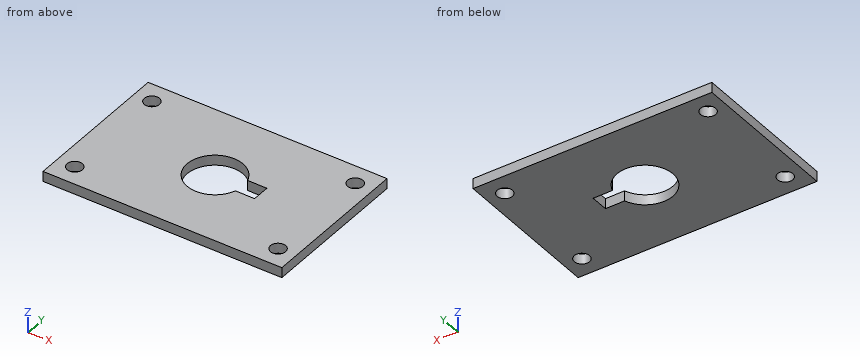
from build123d import *

# Parameters (mm, degrees)
SKETCH_1_W          = 47
SKETCH_1_H          = 30
EXTRUDE_1_DEPTH     = 2
SKETCH_2_R          = 5.5
CUT_EXTRUDE_1_DEPTH = 56.794264938
SKETCH_3_W          = 7
SKETCH_3_H          = 3.5
CUT_EXTRUDE_2_DEPTH = 56.794264938
SKETCH_4_R          = 1.5
CUT_EXTRUDE_3_DEPTH = 56.794264938


with BuildPart() as part:
    # Эскиз1 → Бобышка-Вытянуть1 (new body)
    with BuildSketch(Plane.XY):
        with Locations((23.5, 15)):
            Rectangle(SKETCH_1_W, SKETCH_1_H)
    extrude(amount=EXTRUDE_1_DEPTH)

    # Эскиз2 → Вырез-Вытянуть1 (cut, through all)
    with BuildSketch(Plane.XY.offset(2)):
        with Locations((23.5, 15)):
            Circle(SKETCH_2_R)
    extrude(amount=-CUT_EXTRUDE_1_DEPTH, mode=Mode.SUBTRACT)

    # Эскиз3 → Вырез-Вытянуть2 (cut, through all)
    with BuildSketch(Plane.XY.offset(2)):
        with Locations((29, 15)):
            Rectangle(SKETCH_3_W, SKETCH_3_H)
    extrude(amount=-CUT_EXTRUDE_2_DEPTH, mode=Mode.SUBTRACT)

    # Эскиз4 → Вырез-Вытянуть3 (cut, through all)
    with BuildSketch(Plane.XY.offset(2)):
        with Locations((3.5, 4)):
            Circle(SKETCH_4_R)
        with Locations((43.5, 4)):
            Circle(SKETCH_4_R)
        with Locations((43.5, 26)):
            Circle(SKETCH_4_R)
        with Locations((3.5, 26)):
            Circle(SKETCH_4_R)
    extrude(amount=-CUT_EXTRUDE_3_DEPTH, mode=Mode.SUBTRACT)


solid = part.part
CAD build for the part. Positions are in the model's coordinates, mm. Coordinates: 2 decimals unless noted, no trailing zeros. Order: outer loops, then holes, each group sorted by start corner. A loop starts at its lowest first (then second) coordinate and runs counter-clockwise, first axis right, second up.
Item 1: Band-saw the part on A-A on x = 43.5. List the corners of the cut face in (y, z), plus the area to 3 significant figures.
Check sheet entries:
outline: (0, 0) - (2.5, 0) - (2.5, 2) - (0, 2) - close; (5.5, 0) - (24.5, 0) - (24.5, 2) - (5.5, 2) - close; (27.5, 0) - (30, 0) - (30, 2) - (27.5, 2) - close
area: 48.0 mm2
Item 2: Band-saw the part on B-B on y = 4. List the corners of the cut face in (x, z).
Check sheet entries:
outline: (0, 0) - (2, 0) - (2, 2) - (0, 2) - close; (5, 0) - (42, 0) - (42, 2) - (5, 2) - close; (45, 0) - (47, 0) - (47, 2) - (45, 2) - close
Item 3: Band-saw the part on D-D on z = 1.7. List the corners of the cut face in (x, y), plus the area to 3 significant figures.
Check sheet entries:
outline: (0, 0) - (47, 0) - (47, 30) - (0, 30) - close; hole circle Ø3 at (3.5, 4); hole circle Ø3 at (3.5, 26); hole (28.71, 13.25) - (32.5, 13.25) - (32.5, 16.75) - (28.71, 16.75) arc R5.5 ccw (long way) to start; hole circle Ø3 at (43.5, 4); hole circle Ø3 at (43.5, 26)
area: 1,270 mm2
Item 4: Band-saw the part on C-C on x = 23.5. List the corners of the cut face in (y, z).
Check sheet entries:
outline: (0, 0) - (9.5, 0) - (9.5, 2) - (0, 2) - close; (20.5, 0) - (30, 0) - (30, 2) - (20.5, 2) - close
Item 5: Drill centre lines: L1, parallel to Y at x = 43.5, z = 1.3; L2, parallel to Y at x = 2.5, z = 1.45; L3, parallel to Y at x = 29.5, z = 0.75. Where is each one in solid material? Low to high.
Check sheet entries:
L1: y = 0 to 2.5, 5.5 to 24.5, 27.5 to 30
L2: y = 0 to 2.88, 5.12 to 24.88, 27.12 to 30
L3: y = 0 to 13.25, 16.75 to 30
